```python
from build123d import *

# Parameters (mm, degrees)
F1_DEPTH = 76.2
F3_D     = 6.35
F4_W     = 24.373029
F4_H     = 30.136249
F5_DEPTH = 15.38986


with BuildPart() as f1:
    # F0 (on Front) → F1 (new body)
    with BuildSketch(Plane.XZ):
        Polygon((-64.54286, 51.968571), (-63.009351, 0), (0, 0), (0, -60.967304), (56.001253, -60.967304), (56.001253, 51.968571), align=None)
    extrude(amount=F1_DEPTH)

    # F3 (through all)
    with Locations(Plane(origin=(0, 0, 0), x_dir=(-1, 0, 0), z_dir=(0, 1, 0))):
        with Locations((-40.89044, 38.303375), (-17.421992, 38.303375), (-17.421992, 0), (-40.89044, 0)):
            Hole(F3_D / 2)

    # F4 (on face) → F5 (join)
    with BuildSketch(Plane.XZ.offset(76.2)):
        with Locations((27.447664, -27.442444)):
            Rectangle(F4_W, F4_H)
    extrude(amount=F5_DEPTH)


solid = f1.part
```
Build history of the part. All positions in model axes, mm. A direction names the side the tool comes from. Round coordinates to 2 decimals unless told otherwise and drop trailing zeros. Order: outer loops, then holes, each group sorted by start corner. A loop starts at its lowest first (then second) coordinate and runs counter-clockwise, first axis right, second up. Notation, with made-up numbers: (-26, 85.25) -> (-7, 85.25) arc R12 cw to (-7, 103.25) -> close; hole circle Ø4 at (-4, 31.25). An arc over 180 degrees is marked (long way). Answer in a Markdown table with one row per item.
1) Band-saw the part on D-D on x = -43. Give the cut face in (y, z), and give its area (3 significant figures).
Values:
| item | result |
|---|---|
| outline | (-76.2, 0) -> (0, 0) -> (0, 51.97) -> (-76.2, 51.97) -> close |
| area | 3,960 mm2 |
2) Pin check, flat tips, straight feed: P1, Ø12, axis at x = 17.5, z = -3, coming from the -Y side; P2, Ø12.5, axis at x = 32, y = -86.5, coming from the -Z side; P3, Ø17, axis at y = -84, z = -32, coming from the -X side. Stop position of each tip, or through.
Values:
| item | result |
|---|---|
| P1 | y = -76.2 |
| P2 | z = -42.51 |
| P3 | x = 0 |
3) Band-saw the part on A-A on y = -23. Give the cut face in (x, z) (3 decimals).
Values:
| item | result |
|---|---|
| outline | (-64.543, 51.969) -> (-63.009, 0) -> (0, 0) -> (0, -60.967) -> (56.001, -60.967) -> (56.001, 51.969) -> close; hole circle Ø6.35 at (17.422, 0); hole circle Ø6.35 at (17.422, 38.303); hole circle Ø6.35 at (40.89, 0); hole circle Ø6.35 at (40.89, 38.303) |
4) Band-saw the part on B-B on x = 28. Give the cut face in (y, z).
Values:
| item | result |
|---|---|
| outline | (-91.59, -42.51) -> (-76.2, -42.51) -> (-76.2, -60.97) -> (0, -60.97) -> (0, 51.97) -> (-76.2, 51.97) -> (-76.2, -12.37) -> (-91.59, -12.37) -> close |
5) Wall check: L1, parallel to Z at x = 41, y = -76; L2, parallel to Z at x = 18.5, y = -33; L3, parallel to X at y = -73.5, z = -34. Give the ranges that are in metal, low to high.
Values:
| item | result |
|---|---|
| L1 | -60.97 to -3.17, 3.17 to 35.13, 41.48 to 51.97 |
| L2 | -60.97 to -2.99, 2.99 to 35.32, 41.29 to 51.97 |
| L3 | 0 to 56 |
6) Band-saw the part on C-C on z = -36. Give the cut face in (x, y), and give its area (3 significant figures).
Values:
| item | result |
|---|---|
| outline | (0, -76.2) -> (15.26, -76.2) -> (15.26, -91.59) -> (39.63, -91.59) -> (39.63, -76.2) -> (56, -76.2) -> (56, 0) -> (0, 0) -> close |
| area | 4,640 mm2 |
7) Mould opens along Z. For faces 1 (the flat face through (39.634, -84, -28)), 2 (the cylindrical face through (20.355, -38.633, -1.216)), 3 (the flat face through (27, -84, -12.374)) say: released by +Z, released by -Z, zero draft, split by the parting line, or undercut.
Values:
| item | result |
|---|---|
| face 1 | zero draft |
| face 2 | undercut |
| face 3 | released by +Z |
8) Which spindle directions (+Z, -Z, +X, -X, +Y, -Y) get a long thin tool onto all of the face, cutting with end or side? Do faces 4 (the cylindrical face through (40.202, -38.633, 35.204)), 5 (the flat face through (27, -84, -42.511)), 6 (the flat face through (0, -38, -30)), 7 (the flat face through (15.261, -84, -28)). Say none if no direction does.
Values:
| item | result |
|---|---|
| face 4 | +Y, -Y |
| face 5 | -Z, +X, -X, -Y |
| face 6 | -Z, -X, +Y, -Y |
| face 7 | +Z, -Z, -X, -Y |
